Answer from the drawing. Dimensions are ordinates in mm from the lowest x, y and z of the part. A direction names the side the tool comes from. Round coordinates to 2 decimals unless told otherwise and drop trailing zeros. Write each loop counter-clockwise with the first axis right and the second up, starting at its lowest first coordinate (ties: lowest second). Pieces come first, ordered by that corner, then holes. Notation, with made-up numbers: (40.25, -13) - (54.25, -13) arc R6 cw to (54.25, -7) - close; hole circle Ø10 at (53.5, 21.25). An arc over 180 degrees is marked (long way). Return JSON: item names as keys, results as strings. Group by question number.
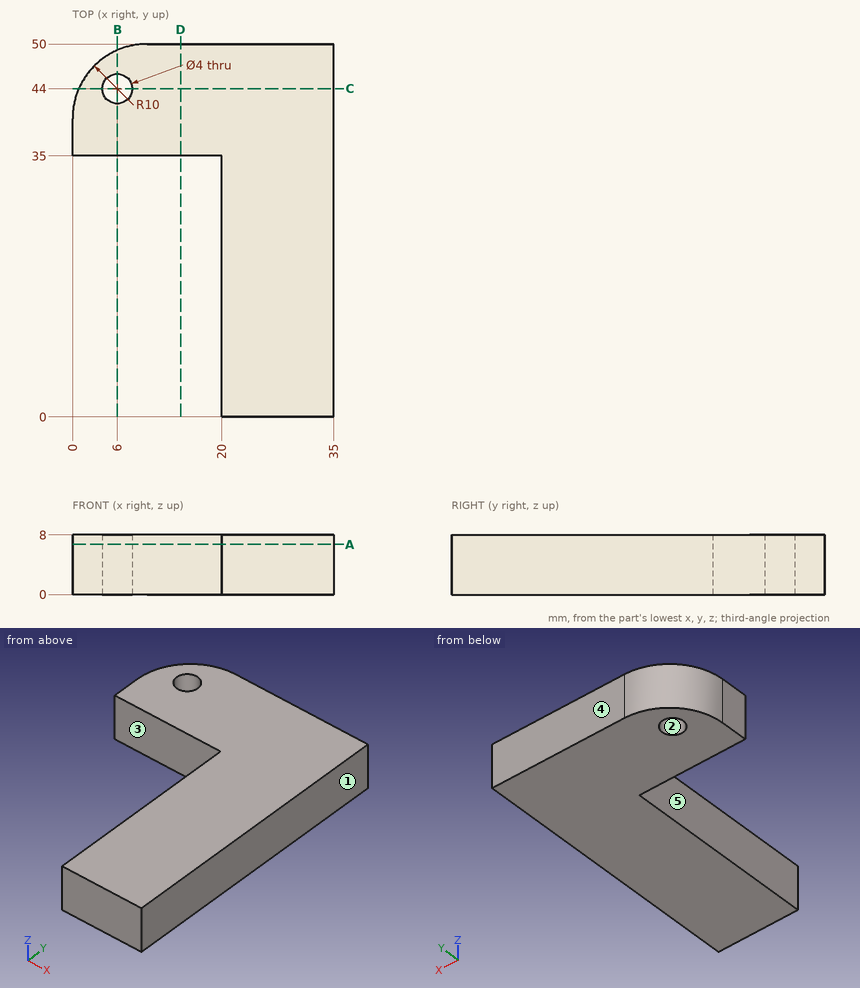
(1) Consider line 1 (X direction, y = 26, z = 1.5); line 2 (X direction, y = 44, z = 4.75); line 3 (Y direction, x = 6, z = 3.75). Determine where each line is inside the solid, lowest interval first.
(2) Determine the mould class of the marked faces 1, 2 and 3 for opening direction Y: +Y half, -Y half, draft (parallel to the pull), parting line (faces both ways), or undercut.
(3) Flat-ended cylindrical pins translate along their axes: pin 1 (4 mm diameter, centred on x = 6, z = 4, fed in from -Y); pin 2 (2 mm diameter, centred on y = 44.5, z = 3, fed in from -X); pin 3 (2.5 mm diameter, centred on x = 6, y = 44, fed in from +Z); pin 4 (5 mm diameter, centred on x = 26, y = 27, fed in from -Z). Find the tip coordinate at first contact, or state that the pin passes through.
(4) Find section C-C (y = 44). Write down the section's boundary in (x, z).
(5) Find section D-D (x = 14.5). Write down the section's boundary in (y, z).
(6) Find section A-A (z = 6.75). Write down the section's boundary in (x, y), plus the area to 3 significant figures.
(7) For the marked faces 4 and 5, determine the directions among +Z, -Z, +X, -X, +Y, -Y from which every point of the face is accessible in a straight line to the end or side of a thin tool.
(8) Find section B-B (x = 6). Write down the section's boundary in (y, z).
Check sheet entries:
{
 "1": {"line 1": "x = 20 to 35", "line 2": "x = 0.83 to 4, 8 to 35", "line 3": "y = 35 to 42, 46 to 49.17"},
 "2": {"face 1": "draft", "face 2": "undercut", "face 3": "-Y half"},
 "3": {"pin 1": "stops at y = 35", "pin 2": "stops at x = 0.63", "pin 3": "passes through", "pin 4": "stops at z = 0"},
 "4": {"outline": "(0.83, 0) - (4, 0) - (4, 8) - (0.83, 8) - close; (8, 0) - (35, 0) - (35, 8) - (8, 8) - close"},
 "5": {"outline": "(35, 0) - (50, 0) - (50, 8) - (35, 8) - close"},
 "6": {"outline": "(0, 35) - (20, 35) - (20, 0) - (35, 0) - (35, 50) - (10, 50) arc R10 ccw to (0, 40) - close; hole circle Ø4 at (6, 44)", "area": "1,020 mm^2"},
 "7": {"face 4": "+Z, -Z, +X, -X, +Y", "face 5": "+Z, -Z, -X, -Y"},
 "8": {"outline": "(35, 0) - (42, 0) - (42, 8) - (35, 8) - close; (46, 0) - (49.17, 0) - (49.17, 8) - (46, 8) - close"}
}
